Here's how the part is built. I have some questions about the finished solid (model axes, mm). A direction names the side the tool comes from. Give positions to 0.01 mm unless a question says otherwise; leave off trailing zeros. Order: outer loops, then holes, each group sorted by start corner. A loop starts at its lowest first (then second) coordinate and runs counter-clockwise, first axis right, second up. Notation, with made-up numbers: (-7.75, 70.5) - (2.25, 70.5) arc R14 cw to (2.25, 80.5) - close; hole circle Ø10 at (39.25, 53). An arc over 180 degrees is marked (long way). One line per question, with ' | ' between items.
from build123d import *

# Parameters (mm, degrees)
SKETCH_1_W      = 150
SKETCH_1_H      = 40
SKETCH_1_R      = 1.6
SKETCH_1_W_2    = 18
SKETCH_1_H_2    = 29.000000001
EXTRUDE_1_DEPTH = 3
FILLET_1_R      = 5


with BuildPart() as part:
    # ｽｹｯﾁ1 → ﾎﾞｽ - 押し出し1 (new body)
    with BuildSketch(Plane(origin=(0, 0, 0), x_dir=(1, 0, 0), z_dir=(0, 1, 0))):
        with Locations((75, 25)):
            Rectangle(SKETCH_1_W, SKETCH_1_H)
        with Locations(Location((143, 25, 0), (0, 0, 90))):
            Circle(SKETCH_1_R, mode=Mode.SUBTRACT)
        with Locations(Location((7, 25, 0), (0, 0, 270))):
            Circle(SKETCH_1_R, mode=Mode.SUBTRACT)
        with Locations((19.999999998, 24.999999999)):
            Rectangle(SKETCH_1_W_2, SKETCH_1_H_2, mode=Mode.SUBTRACT)
        with Locations((40.999999998, 24.999999999)):
            Rectangle(SKETCH_1_W_2, SKETCH_1_H_2, mode=Mode.SUBTRACT)
        with Locations((64.5, 24.999999999)):
            Rectangle(SKETCH_1_W_2, SKETCH_1_H_2, mode=Mode.SUBTRACT)
        with Locations((85.5, 24.999999999)):
            Rectangle(SKETCH_1_W_2, SKETCH_1_H_2, mode=Mode.SUBTRACT)
        with Locations((109.000000002, 24.999999999)):
            Rectangle(SKETCH_1_W_2, SKETCH_1_H_2, mode=Mode.SUBTRACT)
        with Locations((130.000000002, 24.999999999)):
            Rectangle(SKETCH_1_W_2, SKETCH_1_H_2, mode=Mode.SUBTRACT)
    extrude(amount=EXTRUDE_1_DEPTH)

    # ﾌｨﾚｯﾄ1
    fillet_1_edges = [part.edges().sort_by_distance(p)[0] for p in [
        (0, 1.5, -45),
        (150, 1.5, -45),
        (150, 1.5, -5),
        (0, 1.5, -5),
    ]]
    fillet(fillet_1_edges, radius=FILLET_1_R)


solid = part.part
1) I want a section at D-D (x = 7). List the corners of the cut face in (y, z) for me, plus the area to 3 significant figures.
Model answer:
outline: (0, -45) - (3, -45) - (3, -26.6) - (0, -26.6) - close; (0, -23.4) - (3, -23.4) - (3, -5) - (0, -5) - close | area: 110 mm2
2) Thinking about a two-plate mould opening in X: for faces 1 (the face through (0, 1, -25)), 2 (the face through (74, 0, -25)), 3 (the face through (100, 1, -25)), which applies, +X half, -X half, draft (parallel to the pull), parting line (faces both ways), or undercut?
Model answer:
face 1: -X half | face 2: draft | face 3: undercut
3) Please list where these lines run through material, in increasing order: L1, parallel to Z at x = 15, y = 1.75; L2, parallel to Z at x = 143, y = 1.45.
Model answer:
L1: z = -45 to -39.5, -10.5 to -5 | L2: z = -45 to -26.6, -23.4 to -5
4) On a 3-axis mill with a long thin cutter (end or side, diameter ignored), from which of +Z, -Z, +X, -X, +Y, -Y can I reach the whole of each face in a straight line? I mean faces 4 (the face through (74, 3, -25)), 5 (the face through (11, 1, -25)). Say none if no direction works.
Model answer:
face 4: +Z, -Z, +X, -X, +Y | face 5: +Y, -Y
5) I want a section at B-B (y = 1.5). State how many separate pieces and enclosed holes the cut face has, plus the area to 3 significant figures.
Model answer:
separate pieces: 1 | enclosed holes: 8 | area: 2,830 mm2
6) I want a section at C-C (x = 39). List the corners of the cut face in (y, z) for me.
Model answer:
outline: (0, -45) - (3, -45) - (3, -39.5) - (0, -39.5) - close; (0, -10.5) - (3, -10.5) - (3, -5) - (0, -5) - close
7) I want a section at A-A (z = -21). List the corners of the cut face in (x, y) for me, plus the area to 3 significant figures.
Model answer:
outline: (0, 0) - (11, 0) - (11, 3) - (0, 3) - close; (29, 0) - (32, 0) - (32, 3) - (29, 3) - close; (50, 0) - (55.5, 0) - (55.5, 3) - (50, 3) - close; (73.5, 0) - (76.5, 0) - (76.5, 3) - (73.5, 3) - close; (94.5, 0) - (100, 0) - (100, 3) - (94.5, 3) - close; (118, 0) - (121, 0) - (121, 3) - (118, 3) - close; (139, 0) - (150, 0) - (150, 3) - (139, 3) - close | area: 126 mm2
